from build123d import *

# Parameters (mm, degrees)
BOSS_EXTRUDE1_DEPTH = 150
SKETCH2_W           = 336.422734183
SKETCH2_H           = 300
BOSS_EXTRUDE2_DEPTH = 37


with BuildPart() as part:
    # Sketch1 → Boss-Extrude1 (new, symmetric)
    with BuildSketch(Plane(origin=(0, 0, 0), x_dir=(1, 0, 0), z_dir=(0, 1, 0))):
        Polygon((131.503336753, 178.212463787), (146.503336753, 178.212463787), (146.503336753, 201.212463787), (66.503336753, 201.212463787), (66.503336753, 178.212463787), (81.503336753, 178.212463787), (81.503336753, 171.212463787), (59.503336753, 171.212463787), (59.503336753, 208.212463787), (153.503336753, 208.212463787), (153.503336753, 171.212463787), (131.503336753, 171.212463787), align=None)
    extrude(amount=BOSS_EXTRUDE1_DEPTH, both=True)

    # Sketch2 → Boss-Extrude2 (add)
    with BuildSketch(Plane.XY.offset(-171.212463787)):
        with Locations((-108.708030338, 0)):
            Rectangle(SKETCH2_W, SKETCH2_H)
    extrude(amount=-BOSS_EXTRUDE2_DEPTH)


solid = part.part
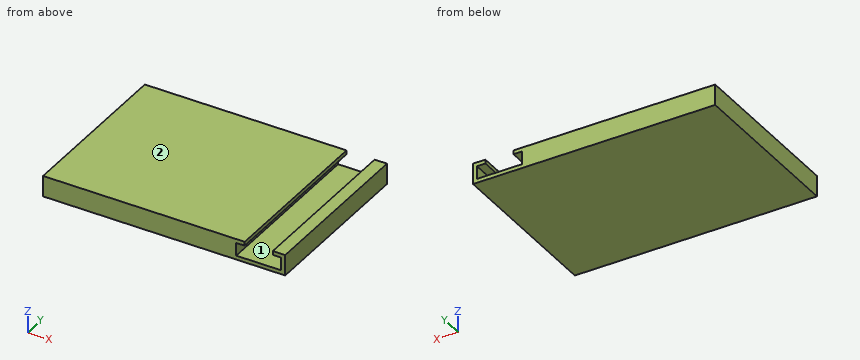
Geometry check sheet. Reference: the model listing, model coordinates, mm. Face numbers are marked on the shaded views. Give positions to 0.01 mm unless a question says otherwise; leave off trailing zeros. Loops run counter-clockwise (first coordinate to the right, second up) from the corner with the lowest first, then second, coordinate; pieces in that order, holes last. Notation, with made-up numbers: M -4,-40 L 51,-40 A18 cw 51,-35 Z; hole C 57,58 d8. An arc over 180 degrees is marked long. Answer as a JSON object with one key per item and string values. Group by question number.
Item 1: Material ranges on L1, parallel to X at y = 29.5, z = -182; L2, parallel to X at y = 42, z = -173; L3, parallel to Z at x = 131, y = -20, recorded low to high.
Item 2: Sectioned sample at B-B on y = -87. Record the boundary of the cut face in (x, z), plus the area to 3 significant figures.
Item 3: Sectioned sample at A-A on z = -196. Record the boundary of the cut face in (x, y), plus the area to 3 significant figures.
Item 4: Sectioned sample at C-C on x = 71.5. Record the boundary of the cut face in (y, z), plus the area to 3 significant figures.
Item 5: Mould release check, pull along X, two halves, no side actions. Record for the marked faces 1 and 2: pulls with the +X half, pulls with the -X half, needs draft (parallel to the pull), parting line crosses it, or undercut.
Findings below:
{
 "1": {"L1": "-276.92 to 66.5, 146.5 to 153.5", "L2": "-276.92 to 81.5, 131.5 to 153.5", "L3": "-208.21 to -201.21"},
 "2": {"outline": "M -276.92,-208.21 L 153.5,-208.21 L 153.5,-171.21 L 131.5,-171.21 L 131.5,-178.21 L 146.5,-178.21 L 146.5,-201.21 L 66.5,-201.21 L 66.5,-178.21 L 81.5,-178.21 L 81.5,-171.21 L -276.92,-171.21 Z", "area": "13,700 mm2"},
 "3": {"outline": "M -276.92,-150 L 66.5,-150 L 66.5,150 L -276.92,150 Z; M 146.5,-150 L 153.5,-150 L 153.5,150 L 146.5,150 Z", "area": "105,000 mm2"},
 "4": {"outline": "M -150,-208.21 L 150,-208.21 L 150,-201.21 L -150,-201.21 Z; M -150,-178.21 L 150,-178.21 L 150,-171.21 L -150,-171.21 Z", "area": "4,200 mm2"},
 "5": {"face 1": "undercut", "face 2": "needs draft"}
}
